```python
from build123d import *

# Parameters (mm, degrees)
SKETCH1_W           = 2
SKETCH1_H           = 40
BOSS_EXTRUDE1_DEPTH = 80
SKETCH2_W           = 2
SKETCH2_H           = 34
BOSS_EXTRUDE2_DEPTH = 60
FILLET1_R           = 1
SKETCH3_R           = 2
CUT_EXTRUDE1_DEPTH  = 142.435497666
SKETCH4_R           = 4
CUT_EXTRUDE2_DEPTH  = 142.435497666


with BuildPart() as part:
    # Sketch1 → Boss-Extrude1 (new body)
    with BuildSketch(Plane.XY):
        Rectangle(SKETCH1_W, SKETCH1_H)
    extrude(amount=BOSS_EXTRUDE1_DEPTH)

    # Sketch2 → Boss-Extrude2 (add)
    with BuildSketch(Plane.XY.offset(80)):
        Rectangle(SKETCH2_W, SKETCH2_H)
    extrude(amount=BOSS_EXTRUDE2_DEPTH)

    # Fillet1
    fillet1_edges = [part.edges().sort_by_distance(p)[0] for p in [
        (0, 17, 80),
        (0, -17, 80),
    ]]
    fillet(fillet1_edges, radius=FILLET1_R)

    # Sketch3 → Cut-Extrude1 (cut, through all)
    with BuildSketch(Plane.ZY.offset(1)):
        with Locations((40, 0)):
            Circle(SKETCH3_R)
    extrude(amount=-CUT_EXTRUDE1_DEPTH, mode=Mode.SUBTRACT)

    # Sketch4 → Cut-Extrude2 (cut, through all)
    with BuildSketch(Plane.ZY.offset(1)):
        with Locations((40, 0)):
            Circle(SKETCH4_R)
    extrude(amount=-CUT_EXTRUDE2_DEPTH, mode=Mode.SUBTRACT)


solid = part.part
```
For this review, take the finished solid that the model builds, in its own axes (mm). Give positions to 0.01 mm unless a question says otherwise; leave off trailing zeros. Write each loop counter-clockwise with the first axis right and the second up, starting at its lowest first coordinate (ties: lowest second). Pieces come first, ordered by that corner, then holes. Notation, with made-up numbers: M 84.5,65 L 107.5,65 A17 cw 107.5,81 Z; hole C 39.5,73.5 d6. An arc over 180 degrees is marked long. Answer as a JSON object with one key per item and string values. Group by question number.
Item 1: Consider section B-B on z = 40. Write out the cut boundary in (x, y).
Item 2: Consider section C-C on x = 0.5. Write out the cut boundary in (y, z).
Item 3: For pin 1 Ø0.6 at (x, y) = (0, -19.5) entering from +Z, flat-tipped, find the tip position at first contact; note if it passes through.
Item 4: Draft analysis for pull direction Z (two halves, no side actions). For faces 1 (the flat face through (1, 0, 69)), 2 (the cylindrical face through (0, -2.4, 36.8)), state which applies: +Z half, -Z half, draft (parallel to the pull), parting line (faces both ways), or undercut.
Item 5: Consider section A-A on y = 0. Write out the cut boundary in (x, z).
Item 6: Consider section D-D on z = 98.5. Write out the cut boundary in (x, y), plus the area to 3 significant figures.
Item 7: For probe 1 along Y at (x, z) = (0.2, 40); probe 2 along Y at (x, z) = (-0.4, 122.5); probe 3 along Z at (x, y) = (0.1, 2), list the stretches that pass through material, from the lowest coordinate up. Write a range as [from, to].
Check result:
{
 "1": {"outline": "M -1,-20 L 1,-20 L 1,-4 L -1,-4 Z; M -1,4 L 1,4 L 1,20 L -1,20 Z"},
 "2": {"outline": "M -20,0 L 20,0 L 20,80 L 18,80 A1 cw 17,81 L 17,140 L -17,140 L -17,81 A1 cw -18,80 L -20,80 Z; hole C 0,40 d8"},
 "3": {"pin 1": "stops at z = 80"},
 "4": {"face 1": "draft", "face 2": "undercut"},
 "5": {"outline": "M -1,0 L 1,0 L 1,36 L -1,36 Z; M -1,44 L 1,44 L 1,140 L -1,140 Z"},
 "6": {"outline": "M -1,-17 L 1,-17 L 1,17 L -1,17 Z", "area": "68.0 mm^2"},
 "7": {"probe 1": "y = [-20, -4], [4, 20]", "probe 2": "y = [-17, 17]", "probe 3": "z = [0, 36.54], [43.46, 140]"}
}
